from build123d import *


with BuildPart() as part:
    # Sketch → Revolution (revolve)
    with BuildSketch(Plane.XZ):
        with BuildLine():
            Line((0.085, 6.215), (0.085, 4.715))
            Line((0.085, 4.715), (0.6, 4.715))
            Line((0.6, 4.715), (0.6, 6.215))
            Line((0.6, 6.215), (0.7, 6.215))
            Line((0.7, 6.215), (0.7, 5.715))
            Line((0.7, 5.715), (1, 5.715))
            Line((1, 5.715), (1, 4.715))
            Line((1, 4.715), (12, 4.715))
            Line((12, 4.715), (12, 0))
            Line((12, 0), (0, 0))
            Line((0, 0), (0, 6.3))
            ThreePointArc((0.085, 6.215), (0.060104, 6.275104), (0, 6.3))
        make_face()
    revolve(axis=Axis((0, 0, 0), (0, 0, 1)))


solid = part.part
Work out the finished part from the listing and answer in its coordinate system (mm). Round coordinates to 2 decimals unless told otherwise and drop trailing zeros. Write each loop counter-clockwise with the first axis right and the second up, starting at its lowest first coordinate (ties: lowest second). Pieces come first, ordered by that corner, then holes.
1) Given pin 1 Ø1.6 at (x, y) = (-0.5, 0.5) entering from +Z, flat-ended and moving along its own axis, determine where the tip first touches the part or whether it passes through.
2) Straight lines are drawn through the part: line 1 (Y direction, x = 0, z = 5.35) (3 decimals); line 2 (Z direction, x = -3.75, y = -0.5) (3 decimals); line 3 (Y direction, x = 0, z = 1.5). For each, find the intervals that lie inside material, in ascending order.
3) A cutting plane is placed at A-A (z = 1.25). Give the vertices of the cut face in (x, y), plus the area to 3 significant figures.
4) The mould has two halves that part along X. Classify faces 1 (the flat face through (-2, 0, 4.715)), 2 (the cylindrical face through (0, -1, 5)), 3 (the cylindrical face through (0.323, 0.506, 5.476)): pulls with the +X half, pulls with the -X half, needs draft (parallel to the pull), parting line crosses it, or undercut.
5) A cutting plane is placed at B-B (x = -4). Give the vertices of the cut face in (y, z) (3 decimals).
6) A cutting plane is placed at C-C (y = 2.75). Give the vertices of the cut face in (x, z) (3 decimals).
Completed:
1. pin 1: stops at z = 6.3
2. line 1: y = -1 to -0.6, -0.085 to 0.085, 0.6 to 1
2. line 2: z = 0 to 4.715
2. line 3: y = -12 to 12
3. outline: circle Ø24 at (0, 0)
3. area: 452 mm2
4. face 1: needs draft
4. face 2: parting line crosses it
4. face 3: undercut
5. outline: (-11.314, 0) - (11.314, 0) - (11.314, 4.715) - (-11.314, 4.715) - close
6. outline: (-11.681, 0) - (11.681, 0) - (11.681, 4.715) - (-11.681, 4.715) - close
